from build123d import *

# Parameters (mm, degrees)
F0_R     = 6.35
F0_R_2   = 1.9939
F1_DEPTH = 4.953
F2_R     = 3.048
F2_R_2   = 1.9939
F3_DEPTH = 0.127
F4_R     = 0.381


with BuildPart() as f1:
    # F0 (on Top) → F1 (new body)
    with BuildSketch(Plane.XY):
        Circle(F0_R)
        Circle(F0_R_2, mode=Mode.SUBTRACT)
    extrude(amount=F1_DEPTH)

    # F2 (on face) → F3 (join)
    with BuildSketch(Plane.XY.offset(4.953)):
        Circle(F2_R)
        Circle(F2_R_2, mode=Mode.SUBTRACT)
    extrude(amount=F3_DEPTH)

    # F4
    f4_edges = [f1.edges().sort_by_distance(p)[0] for p in [
        (-6.35, 0, 4.953),
        (-6.35, 0, 0),
    ]]
    fillet(f4_edges, radius=F4_R)


solid = f1.part
Read the model definition and answer for the solid it produces. Units are mm, in the model's axes. A direction names the side the tool comes from. Give positions to 0.01 mm unless a question says otherwise; leave off trailing zeros. Write each loop counter-clockwise with the first axis right and the second up, starting at its lowest first coordinate (ties: lowest second). Pieces come first, ordered by that corner, then holes. Notation, with made-up numbers: (43.5, 19) - (48.5, 19) arc R14 ccw to (48.5, 29) - close; hole circle Ø9 at (5.5, 67). An arc over 180 degrees is marked (long way). Use CSV: the item, a comma, the result in double quotes. Start each with the question number.
(1) Find section C-C (z = 3.45). Give the vertices of the cut face in (x, y).
(2) Determine the mould class of faces 3 (the cylindrical face through (1.9, 0.6, 2.5)), 4 (the cylindrical face through (-1.38, -6.2, 2.45)), 5 (the flat face through (2, -1, 5.08)) for opening direction X: +X half, -X half, draft (parallel to the pull), parting line (faces both ways), or undercut.
(3) Consider line 1 along Y through (x, z) = (0, 3.1); line 2 along Z through (x, y) = (-4, -2); line 3 along Y through (x, z) = (1.5, 2.05). Determine where each line is inside the solid, lowest interval first.
(4) Given P1, Ø1.5, axis at x = 2.5, z = 2, coming from the -Y side; P2, Ø1.5, axis at y = 3, z = 1, coming from the -X side; P3, Ø2.5, axis at x = 0, y = 0, coming from the +Z side, each flat-ended and moving along its own axis, determine where each tip first touches the part or whether it passes through.
(5) For faces 1 (the flat face through (3, -3, 4.953)), 2 (the flat face through (3, 0, 0)), determine the directions among +Z, -Z, +X, -X, +Y, -Y from which every point of the face is accessible in a straight line to the end or side of a thin tool.
(6) Find section A-A (x = 0). Give the vertices of the cut face in (y, z).
Findings below:
1,outline,"circle Ø12.7 at (0, 0); hole circle Ø3.99 at (0, 0)"
2,face 3,"undercut"
2,face 4,"parting line"
2,face 5,"draft"
3,line 1,"-6.35 to -1.99, 1.99 to 6.35"
3,line 2,"0 to 4.95"
3,line 3,"-6.17 to -1.31, 1.31 to 6.17"
4,P1,"y = -6.1"
4,P2,"x = -5.94"
4,P3,"through"
5,face 1,"+Z"
5,face 2,"-Z, +X, -X, +Y, -Y"
6,outline,"(-6.35, 0.38) arc R0.38 ccw to (-5.97, 0) - (-1.99, 0) - (-1.99, 5.08) - (-3.05, 5.08) - (-3.05, 4.95) - (-5.97, 4.95) arc R0.38 ccw to (-6.35, 4.57) - close; (1.99, 0) - (5.97, 0) arc R0.38 ccw to (6.35, 0.38) - (6.35, 4.57) arc R0.38 ccw to (5.97, 4.95) - (3.05, 4.95) - (3.05, 5.08) - (1.99, 5.08) - close"
